Part model, mm, in its own coordinate system. Round coordinates to 2 decimals unless told otherwise and drop trailing zeros. Write each loop counter-clockwise with the first axis right and the second up, starting at its lowest first coordinate (ties: lowest second). Pieces come first, ordered by that corner, then holes. Notation, with made-up numbers: M 78.25,-12 L 99.25,-12 A6 cw 99.25,-1 Z; hole C -6,67.5 d2. An arc over 180 degrees is marked long. Answer as a JSON object with one key per item and string values. Group by question number.
1. Band-saw the part on D-D, the plane z = 0.5. Write the cut outline in (x, y).
2. Band-saw the part on C-C, the plane x = 0.7. Write the cut outline in (y, z).
3. Band-saw the part on A-A, the plane z = -0.75. Write the cut outline in (x, y), plus the area to 3 significant figures.
4. Drill centre lines: line 1 (Y direction, x = 1.5, z = 6.25); line 2 (Z direction, x = 0.15, y = 1.85). Where is each one in solid material? Low to high. Write a range as from..to.
5. Band-saw the part on B-B, the plane y = 1.55. Write the cut outline in (x, z).
6. Drop a flat-ended pin along its axis: pin 1 (1.5 mm diameter, centred on x = 1.5, y = 1, fed in from +Z). Give the stop position or say it passes through.
from build123d import *

# Parameters (mm, degrees)
SKETCH_2_W          = 2.54
SKETCH_2_H          = 2.54
EXTRUDE_1_DEPTH     = 2.54
FILLET_1_R          = 0.508
EXTRUDE_2_DEPTH     = 7.366
CUT_EXTRUDE_1_DEPTH = 8.96463163
CUT_EXTRUDE_3_DEPTH = 8.96463163


with BuildPart() as part:
    # 草图2 → 凸台-拉伸1 (new body)
    with BuildSketch(Plane.XY):
        with Locations((1.27, 1.27)):
            Rectangle(SKETCH_2_W, SKETCH_2_H)
    extrude(amount=-EXTRUDE_1_DEPTH)

    # 圆角1
    fillet_1_edges = [part.edges().sort_by_distance(p)[0] for p in [
        (0, 2.54, -1.27),
        (2.54, 2.54, -1.27),
        (2.54, 0, -1.27),
        (0, 0, -1.27),
    ]]
    fillet(fillet_1_edges, radius=FILLET_1_R)

    # 草图3 → 凸台-拉伸2 (add)
    with BuildSketch(Plane.XY):
        Polygon((1.651, 1.27), (1.651, 1.651), (0.889, 1.651), (0.889, 0.889), (1.651, 0.889), align=None)
    extrude(amount=EXTRUDE_2_DEPTH)

    # 草图4 → 切除-拉伸1 (cut, through all)
    with BuildSketch(Plane(origin=(1.651, 0, 0), x_dir=(0, 0, -1), z_dir=(1, 0, 0))):
        Polygon((-7.366, 0.889), (-7.366, 1.143), (-7.112, 0.889), align=None)
        Polygon((-7.366, 1.397), (-7.112, 1.651), (-7.366, 1.651), align=None)
    extrude(amount=-CUT_EXTRUDE_1_DEPTH, mode=Mode.SUBTRACT)

    # 草图6 → 切除-拉伸3 (cut, through all)
    with BuildSketch(Plane(origin=(0, 0.889, 0), x_dir=(-1, 0, 0), z_dir=(0, -1, 0))):
        Polygon((-1.143, -7.366), (-0.889, -7.112), (-0.889, -7.366), align=None)
        Polygon((-1.651, -7.366), (-1.397, -7.366), (-1.651, -7.112), align=None)
    extrude(amount=-CUT_EXTRUDE_3_DEPTH, mode=Mode.SUBTRACT)


solid = part.part
Worked answers:
{
 "1": {"outline": "M 0.89,0.89 L 1.65,0.89 L 1.65,1.65 L 0.89,1.65 Z"},
 "2": {"outline": "M 0,-2.54 L 2.54,-2.54 L 2.54,0 L 0,0 Z"},
 "3": {"outline": "M 0,0.51 A0.51 ccw 0.51,0 L 2.03,0 A0.51 ccw 2.54,0.51 L 2.54,2.03 A0.51 ccw 2.03,2.54 L 0.51,2.54 A0.51 ccw 0,2.03 Z", "area": "6.23 mm^2"},
 "4": {"line 1": "y = 0.89..1.65", "line 2": "z = -2.54..0"},
 "5": {"outline": "M 0,-2.54 L 2.54,-2.54 L 2.54,0 L 1.65,0 L 1.65,7.11 L 1.55,7.21 L 0.99,7.21 L 0.89,7.11 L 0.89,0 L 0,0 Z"},
 "6": {"pin 1": "stops at z = 7.37"}
}
